Can you work these out from the drawing? Everything is in mm from the part's minimum corner. Coordinates: 2 decimals unless noted, no trailing zeros. Order: outer loops, then holes, each group sorted by start corner. A loop starts at its lowest first (then second) coordinate and runs counter-clockwise, first axis right, second up. Notation, with made-up numbers: (29, -39) - (73, -39) arc R28 cw to (73, -16) - close; hole circle Ø10 at (37, 70.5). An arc over 180 degrees is marked (long way). Use a Markdown table: item, result. Add a question column.
(1) I want a section at A-A (z = 12.5). List the corners of the cut face in (x, y) for me, and give its area (3 significant figures).
(2) I want a section at C-C (x = 93.82). List the corners of the cut face in (y, z) for me, and give its area (3 significant figures).
(3) I want a section at D-D (y = 120.5). List the corners of the cut face in (x, z) for me, and give its area (3 significant figures).
(4) I want a section at B-B (x = 206). List the corners of the cut face in (y, z) for me.
(5) If I drill on L1, parallel to Y at x = 123.82, z = 10.5 (1 decimal); L2, parallel to X at y = 130, z = 4.5; L3, parallel to Y at x = 93.82, z = 5.25 (1 decimal), over which ranges is the centre line in solid material (lowest first)? Write a range as [from, to].
(6) For pin 1 Ø5 at (y, z) = (230, 4.5) entering from +X; pin 2 Ø4.5 at (y, z) = (97, 6) entering from +X; pin 3 Ø1 at (x, z) = (29.5, 8.5) entering from +Y, each with a flat end and sliding along its axis, tell me the tip position at first contact or that it passes through.
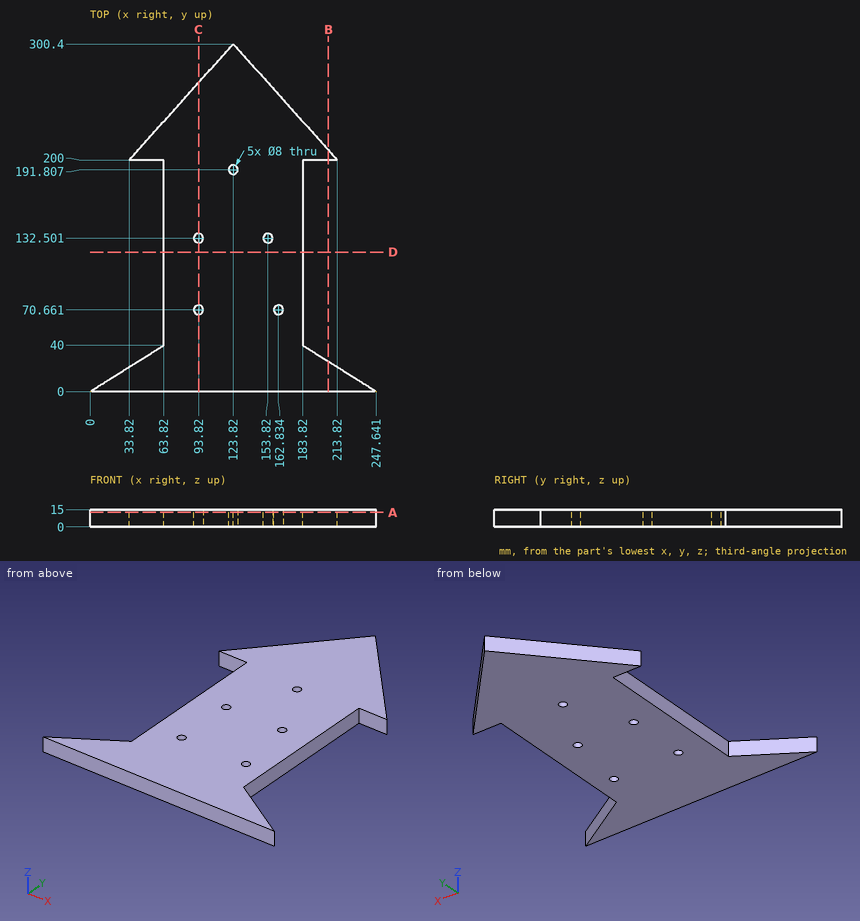
Answers follow:
| question | item | result |
|---|---|---|
| 1 | outline | (0, 0) - (247.64, 0) - (183.82, 40) - (183.82, 200) - (213.82, 200) - (123.82, 300.4) - (33.82, 200) - (63.82, 200) - (63.82, 40) - close; hole circle Ø8 at (93.82, 70.66); hole circle Ø8 at (93.82, 132.5); hole circle Ø8 at (123.82, 191.81); hole circle Ø8 at (153.82, 132.5); hole circle Ø8 at (162.83, 70.66) |
| 1 | area | 35,300 mm² |
| 2 | outline | (0, 0) - (66.66, 0) - (66.66, 15) - (0, 15) - close; (74.66, 0) - (128.5, 0) - (128.5, 15) - (74.66, 15) - close; (136.5, 0) - (266.93, 0) - (266.93, 15) - (136.5, 15) - close |
| 2 | area | 3,760 mm² |
| 3 | outline | (63.82, 0) - (183.82, 0) - (183.82, 15) - (63.82, 15) - close |
| 3 | area | 1,800 mm² |
| 4 | outline | (0, 0) - (26.1, 0) - (26.1, 15) - (0, 15) - close; (200, 0) - (208.72, 0) - (208.72, 15) - (200, 15) - close |
| 5 | L1 | y = [0, 187.8], [195.8, 300.4] |
| 5 | L2 | x = [63.82, 90.7], [96.94, 150.7], [156.94, 183.82] |
| 5 | L3 | y = [0, 66.7], [74.7, 128.5], [136.5, 266.9] |
| 6 | pin 1 | stops at x = 189.17 |
| 6 | pin 2 | stops at x = 183.82 |
| 6 | pin 3 | stops at y = 18.8 |
